Build history of the part. All positions in model axes, mm. Face numbers are marked on the shaded views. A direction names the side the tool comes from. Coordinates: 2 decimals unless noted, no trailing zeros. Write each loop counter-clockwise with the first axis right and the second up, starting at its lowest first coordinate (ties: lowest second). Pieces come first, ordered by that corner, then holes.
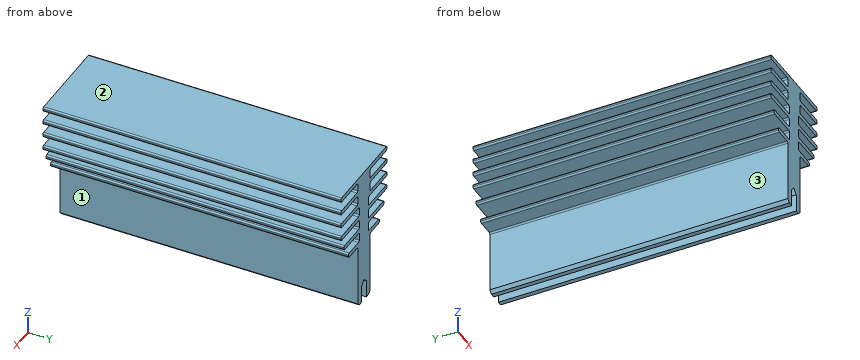
```python
from build123d import *

# Parameters (mm, degrees)
PAD_DEPTH    = 100
FILLET_R     = 0.5
CHAMFER_SIZE = 1


with BuildPart() as part:
    # Sketch → Pad (new body)
    with BuildSketch(Plane.XZ):
        Polygon((0, 7.5), (-1.5, 6), (-1.5, 0), (-4, 0), (-4, 22), (-10, 22), (-10, 23.5), (-3, 23.5), (-3, 26.74), (-13, 26.74), (-13, 28.24), (-3, 28.24), (-3, 31.48), (-15, 31.48), (-15, 32.98), (-3, 32.98), (-3, 36.22), (-15, 36.22), (-15, 37.72), (-4, 37.72), (-4, 40.96), (-15, 40.96), (-15, 42.46), (-4, 42.46), (-4, 45.7), (-15, 45.7), (-15, 47.2), (0, 47.2), (15, 47.2), (15, 45.7), (4, 45.7), (4, 42.46), (15, 42.46), (15, 40.96), (4, 40.96), (4, 37.72), (15, 37.72), (15, 36.22), (3, 36.22), (3, 32.98), (15, 32.98), (15, 31.48), (3, 31.48), (3, 28.24), (13, 28.24), (13, 26.74), (3, 26.74), (3, 23.5), (10, 23.5), (10, 22), (4, 22), (4, 0), (1.5, 0), (1.5, 6.000001), align=None)
    extrude(amount=PAD_DEPTH)

    # Fillet
    fillet_edges = [part.edges().sort_by_distance(p)[0] for p in [
        (3, -50, 28.24),
        (3, -50, 32.98),
        (4, -50, 37.72),
        (4, -50, 42.46),
        (3, -50, 23.5),
        (15, -50, 31.48),
        (13, -50, 26.74),
        (13, -50, 28.24),
        (15, -50, 32.98),
        (15, -50, 36.22),
        (15, -50, 37.72),
        (15, -50, 40.96),
        (15, -50, 42.46),
        (15, -50, 45.7),
        (15, -50, 47.2),
        (10, -50, 22),
        (10, -50, 23.5),
        (4, -50, 22),
        (3, -50, 26.74),
        (3, -50, 31.48),
        (3, -50, 36.22),
        (4, -50, 40.96),
        (4, -50, 45.7),
        (-4, -50, 22),
        (-10, -50, 22),
        (-10, -50, 23.5),
        (-3, -50, 26.74),
        (-13, -50, 26.74),
        (-13, -50, 28.24),
        (-3, -50, 31.48),
        (-15, -50, 31.48),
        (-15, -50, 32.98),
        (-3, -50, 36.22),
        (-15, -50, 36.22),
        (-15, -50, 37.72),
        (-4, -50, 40.96),
        (-15, -50, 40.96),
        (-15, -50, 42.46),
        (-4, -50, 45.7),
        (-15, -50, 45.7),
        (-15, -50, 47.2),
    ]]
    fillet(fillet_edges, radius=FILLET_R)

    # Chamfer
    chamfer_edges = [part.edges().sort_by_distance(p)[0] for p in [
        (4, -50, 0),
        (-4, -50, 0),
    ]]
    chamfer(chamfer_edges, length=CHAMFER_SIZE)


solid = part.part
```
1. Saw through at B-B on z = 10. List the corners of the cut face in (x, y).
Computed values:
outline: (-4, -100) - (4, -100) - (4, 0) - (-4, 0) - close
2. 3-axis set-ups, long thin cutter, end or side, ignore diameter. For the marked faces 1, 2 and 3: which of +Z, -Z, +X, -X, +Y, -Y reach the whole face in a straight line?
Computed values:
face 1: -Z, +X, +Y, -Y
face 2: +Z, +X, -X, +Y, -Y
face 3: -Z, -X, +Y, -Y
3. Flat gauge pins, fed straight in: pin 1 (6 mm diameter, centred on y = -41.5, z = 16, fed in from -X); pin 2 (3 mm diameter, centred on x = -6.5, y = -37, fed in from -Z); pin 3 (2.5 mm diameter, centred on y = -39.5, z = 39.5, fed in from +X); pin 4 (12 mm diameter, centred on x = -3, z = 39, fed in from +Y). Where does each tip first touch, or does it go through?
Computed values:
pin 1: stops at x = -4
pin 2: stops at z = 22
pin 3: stops at x = 4.09
pin 4: stops at y = 0
4. Probe line 1 along Z through (x, y) = (8.75, -6.5); line 2 along Z through (x, y) = (12.5, -12); line 3 along Z through (x, y) = (13.75, -49). List the from-to ranges inside material, lowest first.
Computed values:
line 1: z = 22 to 23.5, 26.74 to 28.24, 31.48 to 32.98, 36.22 to 37.72, 40.96 to 42.46, 45.7 to 47.2
line 2: z = 26.74 to 28.24, 31.48 to 32.98, 36.22 to 37.72, 40.96 to 42.46, 45.7 to 47.2
line 3: z = 31.48 to 32.98, 36.22 to 37.72, 40.96 to 42.46, 45.7 to 47.2
5. Saw through at A-A on x = -6.75. List the corners of the cut face in (y, z).
Computed values:
outline: (-100, 22) - (0, 22) - (0, 23.5) - (-100, 23.5) - close; (-100, 26.74) - (0, 26.74) - (0, 28.24) - (-100, 28.24) - close; (-100, 31.48) - (0, 31.48) - (0, 32.98) - (-100, 32.98) - close; (-100, 36.22) - (0, 36.22) - (0, 37.72) - (-100, 37.72) - close; (-100, 40.96) - (0, 40.96) - (0, 42.46) - (-100, 42.46) - close; (-100, 45.7) - (0, 45.7) - (0, 47.2) - (-100, 47.2) - close
